from build123d import *

# Parameters (mm, degrees)
ESQUISSE2_W        = 406.6
ESQUISSE2_H        = 177.8
ESQUISSE2_R        = 12
ESQUISSE2_R_2      = 15
BOSS_EXTRU_3_DEPTH = 30
ESQUISSE4_W        = 406.6
ESQUISSE4_H        = 177.8
BOSS_EXTRU_4_DEPTH = 4


with BuildPart() as part:
    # Esquisse2 → Boss.-Extru.3 (new body)
    with BuildSketch(Plane.XY):
        with Locations((203.3, 88.9)):
            Rectangle(ESQUISSE2_W, ESQUISSE2_H)
        with Locations((134.07925081, 115.620543461)):
            Circle(ESQUISSE2_R, mode=Mode.SUBTRACT)
        with Locations((163.619308258, 115.709309955)):
            Circle(ESQUISSE2_R, mode=Mode.SUBTRACT)
        with Locations((189.931391461, 102.812951429)):
            Circle(ESQUISSE2_R, mode=Mode.SUBTRACT)
        with Locations((215.148770887, 85.431045161)):
            Circle(ESQUISSE2_R, mode=Mode.SUBTRACT)
        with Locations((205.406615555, 50.360364433)):
            Circle(ESQUISSE2_R_2, mode=Mode.SUBTRACT)
        with Locations((217.770290506, 114.829364891)):
            Circle(ESQUISSE2_R, mode=Mode.SUBTRACT)
        with Locations((244.688210229, 126.551247272)):
            Circle(ESQUISSE2_R, mode=Mode.SUBTRACT)
        with Locations((274.33036562, 125.743518948)):
            Circle(ESQUISSE2_R, mode=Mode.SUBTRACT)
        with Locations((303.876863168, 122.656060434)):
            Circle(ESQUISSE2_R, mode=Mode.SUBTRACT)
        with Locations((303.54762398, 91.701693193)):
            Circle(ESQUISSE2_R, mode=Mode.SUBTRACT)
        with Locations((274.160623302, 96.722519891)):
            Circle(ESQUISSE2_R, mode=Mode.SUBTRACT)
        with Locations((243.010025324, 96.447343803)):
            Circle(ESQUISSE2_R, mode=Mode.SUBTRACT)
    extrude(amount=BOSS_EXTRU_3_DEPTH)

    # Esquisse4 → Boss.-Extru.4 (add)
    with BuildSketch(Plane(origin=(0, 0, 0), x_dir=(-1, 0, 0), z_dir=(0, 0, -1))):
        with Locations((-203.3, 88.9)):
            Rectangle(ESQUISSE4_W, ESQUISSE4_H)
    extrude(amount=-BOSS_EXTRU_4_DEPTH)


solid = part.part
Read the model definition and answer for the solid it produces. Units are mm, in the model's axes. A direction names the side the tool comes from. Round coordinates to 2 decimals unless told otherwise and drop trailing zeros. Loops run counter-clockwise (first coordinate to the right, second up) from the corner with the lowest first, then second, coordinate; pieces in that order, holes last.
Q1. Section D-D on x = 243 is taken. Write down the section's boundary in (y, z).
Q2. This flat-tipped pin is pushed along its axis until it touches: pin 1 (12 mm diameter, centred on x = 135.5, y = 118, fed in from +Z). Where does it stop, or does it pass through?
Q3. Section A-A on z = 19.5 is taken. Give the number of separate pieces and of enclosed holes in the cut face, and give its area (3 significant figures).
Q4. Determine the mould class of faces 3 (the face through (200, 0, 15)), 4 (the face through (0, 88, 15)), 5 (the face through (243.13, 138.45, 16.82)), 6 (the face through (280.781, 135.862, 16.818)) for opening direction X: released by +X, released by -X, zero draft, split by the parting line, or undercut.
Q5. Consider probe 1 along X at (y, z) = (87, 19.5); probe 2 along X at (y, z) = (135.5, 24); probe 3 along X at (y, z) = (86.5, 18.5). Determine where each line is inside the solid, lowest interval first.
Q6. Which of the six approach directions +Z, -Z, +X, -X, +Y, -Y give full straight-line access (tool end or side, diameter ignored) to faces 1 (the face through (200, 177.8, 15)), 2 (the face through (134, 116, 4))?
Q7. Section C-C on x = 310 is taken. Write down the section's boundary in (y, z).
Q8. Section B-B on y = 61.5 is taken. Write down the section's boundary in (x, z).
Output:
1. outline: (0, 0) - (177.8, 0) - (177.8, 30) - (138.43, 30) - (138.43, 4) - (114.67, 4) - (114.67, 30) - (108.45, 30) - (108.45, 4) - (84.45, 4) - (84.45, 30) - (0, 30) - close
2. pin 1: stops at z = 4
3. separate pieces: 1
3. enclosed holes: 12
3. area: 66,600 mm2
4. face 3: zero draft
4. face 4: released by -X
4. face 5: undercut
4. face 6: undercut
5. probe 1: x = 0 to 203.25, 227.05 to 235.61, 250.41 to 267.13, 281.19 to 292.51, 314.59 to 406.6
5. probe 2: x = 0 to 236.69, 252.68 to 267.34, 281.32 to 406.6
5. probe 3: x = 0 to 203.2, 227.1 to 236.3, 249.72 to 267.88, 280.45 to 292.73, 314.36 to 406.6
6. face 1: +Z, -Z, +X, -X, +Y
6. face 2: +Z
7. outline: (0, 0) - (177.8, 0) - (177.8, 30) - (132.98, 30) - (132.98, 4) - (112.34, 4) - (112.34, 30) - (101.82, 30) - (101.82, 4) - (81.58, 4) - (81.58, 30) - (0, 30) - close
8. outline: (0, 0) - (406.6, 0) - (406.6, 30) - (215.45, 30) - (215.45, 4) - (195.36, 4) - (195.36, 30) - (0, 30) - close
